Autodesk Inventor part; units mm, degrees
ref_plane "YZ Plane" through (0, 0, 0) normal (1, 0, 0) x (0, 1, 0)
ref_plane "XZ Plane" through (0, 0, 0) normal (0, 1, 0) x (-1, 0, 0)
ref_plane "XY Plane" through (0, 0, 0) normal (0, 0, 1) x (1, 0, 0)
sketch "Sketch1" plane through (0, 0, 0) normal (0, 0, 1) x (1, 0, 0)
  line L0 (13.5, -13.5) -> (-13.5, -13.5)
  line L1 (-13.5, -13.5) -> (-13.5, 13.5)
  line L2 (-13.5, 13.5) -> (13.5, 13.5)
  line L3 (13.5, 13.5) -> (13.5, -13.5)
  line L4 (13.5, -13.5) -> (-13.5, 13.5) construction
  line L5 (-13.5, -13.5) -> (13.5, 13.5) construction
  point P0 (0, 0)
  dimension "d0" = 27
extrude "Extrusion1" add sketch "Sketch1" along normal mid plane 0.56
sketch "Sketch2" plane through (0, 0, 0.28) normal (0, 0, 1) x (1, 0, 0)
  line L0 (-13.5, -13.5) -> (13.5, -13.5)
  line L1 (13.5, -13.5) -> (13.5, 13.5)
  line L2 (0, 0) -> (0, -13.5)
  line L3 (0, 0) -> (13.5, 0)
  point P0 (10.2, -10.2)
  dimension "d3" = 20.4
  dimension "d4" = 20.4
hole "Hole1" at (10.2, -10.2, 0.28) direction (0, 0, -1) diameter 2.5 end through all
pattern_circular "Circular Pattern1" count 4 over 360 about axis through (0, 0, -10) along (0, 0, 1) of "Hole1"
sketch "Sketch3" plane through (0, 0, 0.28) normal (0, 0, 1) x (1, 0, 0)
  circle A0 centre (-3.52, 8.5) radius 1
  point P0 (0, 0)
  dimension "d15" = 2
  dimension "d16" = 3.52
  dimension "d17" = 8.5
extrude "Extrusion2" cut sketch "Sketch3" against normal through all
mirror "Mirror1" about plane through (0, 0, 0) normal (1, 0, 0) of "Extrusion2"
pattern_circular "Circular Pattern2" count 4 over 360 about axis through (0, 0, -10) along (0, 0, 1) of "Extrusion2", "Mirror1"
ref_plane "Work Plane1" through (-3.52, 8.5, 0.28) normal (-0.9239, -0.3826, 0) x (0, 0, -1)
sketch "Sketch4" plane through (0, 0, 0.28) normal (0, 0, 1) x (1, 0, 0)
  line L0 (-4.0305, 0) -> (0, 4.0305)
  line L1 (0, 4.0305) -> (4.0305, 0)
  line L2 (4.0305, 0) -> (0, -4.0305)
  line L3 (0, -4.0305) -> (-4.0305, 0)
  line L4 (0, 4.0305) -> (0, -4.0305) construction
  line L5 (-4.0305, 0) -> (4.0305, 0) construction
  point P0 (0, 0)
  point P1 (0, 0)
  dimension "d23" = 5.7
extrude "Extrusion3" add sketch "Sketch4" along normal blind 0.1
properties part number "PCB"
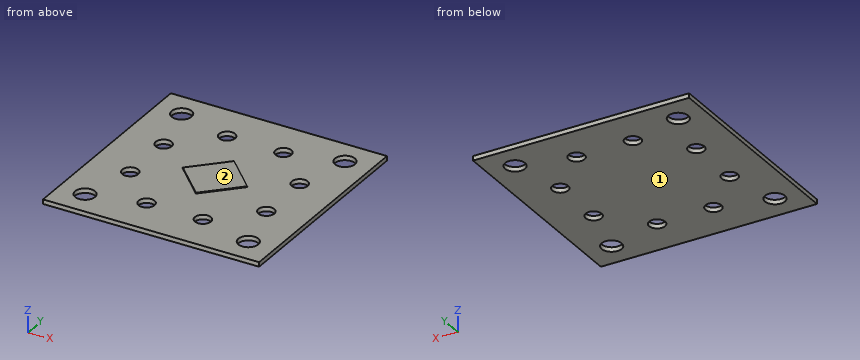
Here's how the part is built. I have some questions about the finished solid (model axes, mm). Face numbers are marked on the shaded views. Coordinates: 2 decimals unless noted, no trailing zeros. Loops run counter-clockwise (first coordinate to the right, second up) from the corner with the lowest first, then second, coordinate; pieces in that order, holes last. Notation, with made-up numbers: (22.5, 9) - (60.5, 9) arc R12 ccw to (60.5, 32) - close; hole circle Ø4 at (84, 65.5). An arc over 180 degrees is marked (long way). Return JSON: item names as keys, results as strings. Group by question number.
Item 1: If we section it at A-A on x = 10.2: Write out the boundary of the cut face in (y, z), and give its area (3 significant figures).
Item 2: If we section it at B-B on z = -0.1: State how many separate pieces and enclosed holes the cut face has, and give its area (3 significant figures).
Item 3: Will these pins go through, and if not, where does the flat tip stop? P1, Ø1.5, axis at x = -10.2, y = 10.2, coming from the +Z side (3 decimals); P2, Ø1, axis at x = 10.5, y = -8, coming from the +Z side; P3, Ø2.5, axis at x = -8.5, y = -3.52, coming from the -Z side.
Item 4: If we section it at C-C on y = -8.5: Write out the boundary of the cut face in (x, z).
Item 5: If we section it at D-D on y = 3.52: Write out the boundary of the cut face in (x, z).
Item 6: We'd pull the mould along Z, two halves only. Please class the marked faces 1 and 2: +Z half, -Z half, draft (parallel to the pull), parting line (faces both ways), or undercut.
Item 7: I need wall thicknesses on line 1 (Y direction, x = -3.52, z = 0); line 2 (Y direction, x = -8.5, z = 0); line 3 (X direction, y = 8, z = 0.2). Which ranges of each line are inside material? Lowest first, please. Write a range as from..to.
Calculated:
{
 "1": {"outline": "(-13.5, -0.28) - (-11.45, -0.28) - (-11.45, 0.28) - (-13.5, 0.28) - close; (-8.95, -0.28) - (8.95, -0.28) - (8.95, 0.28) - (-8.95, 0.28) - close; (11.45, -0.28) - (13.5, -0.28) - (13.5, 0.28) - (11.45, 0.28) - close", "area": "12.3 mm^2"},
 "2": {"separate pieces": "1", "enclosed holes": "12", "area": "684 mm^2"},
 "3": {"P1": "passes through", "P2": "stops at z = 0.28", "P3": "stops at z = -0.28"},
 "4": {"outline": "(-13.5, -0.28) - (-4.52, -0.28) - (-4.52, 0.28) - (-13.5, 0.28) - close; (-2.52, -0.28) - (2.52, -0.28) - (2.52, 0.28) - (-2.52, 0.28) - close; (4.52, -0.28) - (13.5, -0.28) - (13.5, 0.28) - (4.52, 0.28) - close"},
 "5": {"outline": "(-13.5, -0.28) - (-9.5, -0.28) - (-9.5, 0.28) - (-13.5, 0.28) - close; (-7.5, -0.28) - (7.5, -0.28) - (7.5, 0.28) - (0.51, 0.28) - (0.51, 0.38) - (-0.51, 0.38) - (-0.51, 0.28) - (-7.5, 0.28) - close; (9.5, -0.28) - (13.5, -0.28) - (13.5, 0.28) - (9.5, 0.28) - close"},
 "6": {"face 1": "-Z half", "face 2": "+Z half"},
 "7": {"line 1": "y = -13.5..-9.5, -7.5..7.5, 9.5..13.5", "line 2": "y = -13.5..-4.52, -2.52..2.52, 4.52..13.5", "line 3": "x = -13.5..-4.39, -2.65..2.65, 4.39..13.5"}
}
